Geometry check sheet. Reference: the model listing, model coordinates, mm. Face numbers are marked on the shaded views. A direction names the side the tool comes from. Give positions to 0.01 mm unless a question says otherwise; leave off trailing zeros. Order: outer loops, then holes, each group sorted by start corner. A loop starts at its lowest first (then second) coordinate and runs counter-clockwise, first axis right, second up. Notation, with made-up numbers: M -29.5,72 L -17.5,72 A20 cw -17.5,108 Z; hole C 26.25,-11.5 d3. An arc over 180 degrees is marked long. One line per question, with ' | ' between items. Start each with the question number.
from build123d import *

# Parameters (mm, degrees)
Y_KSEKLIK_EKSTR_ZYON4_DEPTH = 20
IZIM5_R                     = 67.8
IZIM5_R_2                   = 50
KES_EKSTR_ZYON1_DEPTH       = 10
IZIM7_R                     = 50
KES_EKSTR_ZYON2_DEPTH       = 20


with BuildPart() as part:
    # Çizim1 → Yükseklik-Ekstrüzyon4 (new body)
    with BuildSketch(Plane(origin=(0, 0, 0), x_dir=(1, 0, 0), z_dir=(0, 1, 0))):
        with BuildLine():
            ThreePointArc((-141.825379968, 39.155786128), (-171.116823462, 33.971749541), (-188.729833462, 10))
            Line((-188.729833462, 10), (-172.912878475, 10))
            ThreePointArc((-172.912878475, 10), (-125, 0), (-172.912878475, -10))
            Line((-172.912878475, -10), (-188.729833462, -10))
            ThreePointArc((-188.729833462, -10), (-171.116823462, -33.971749541), (-141.825379968, -39.155786128))
            ThreePointArc((-141.825379968, -39.155786128), (-90.896626459, -39.380855183), (-44.495770634, -60.374882159))
            ThreePointArc((-44.495770634, -60.374882159), (0, -75), (44.495770634, -60.374882159))
            ThreePointArc((44.495770634, -60.374882159), (90.896626459, -39.380855183), (141.825379968, -39.155786128))
            ThreePointArc((141.825379968, -39.155786128), (171.116823462, -33.971749541), (188.729833462, -10))
            Line((188.729833462, -10), (172.912878475, -10))
            ThreePointArc((172.912878475, -10), (125, 0), (172.912878475, 10))
            Line((172.912878475, 10), (188.729833462, 10))
            ThreePointArc((188.729833462, 10), (171.116823462, 33.971749541), (141.825379968, 39.155786128))
            ThreePointArc((141.825379968, 39.155786128), (90.896626459, 39.380855183), (44.495770634, 60.374882159))
            ThreePointArc((44.495770634, 60.374882159), (0, 75), (-44.495770634, 60.374882159))
            ThreePointArc((-44.495770634, 60.374882159), (-90.896626459, 39.380855183), (-141.825379968, 39.155786128))
        make_face()
    extrude(amount=Y_KSEKLIK_EKSTR_ZYON4_DEPTH)

    # Çizim5 → Kes-Ekstrüzyon1 (cut)
    with BuildSketch(Plane(origin=(0, 20, 0), x_dir=(1, 0, 0), z_dir=(0, 1, 0))):
        with Locations(Location((0, 0, 0), (0, 0, 270))):
            Circle(IZIM5_R)
        with Locations(Location((0, 0, 0), (0, 0, 270))):
            Circle(IZIM5_R_2, mode=Mode.SUBTRACT)
    extrude(amount=-KES_EKSTR_ZYON1_DEPTH, mode=Mode.SUBTRACT)

    # Çizim7 → Kes-Ekstrüzyon2 (cut)
    with BuildSketch(Plane(origin=(0, 20, 0), x_dir=(1, 0, 0), z_dir=(0, 1, 0))):
        with Locations(Location((0, 0, 0), (0, 0, 270))):
            Circle(IZIM7_R)
    extrude(amount=-KES_EKSTR_ZYON2_DEPTH, mode=Mode.SUBTRACT)


solid = part.part
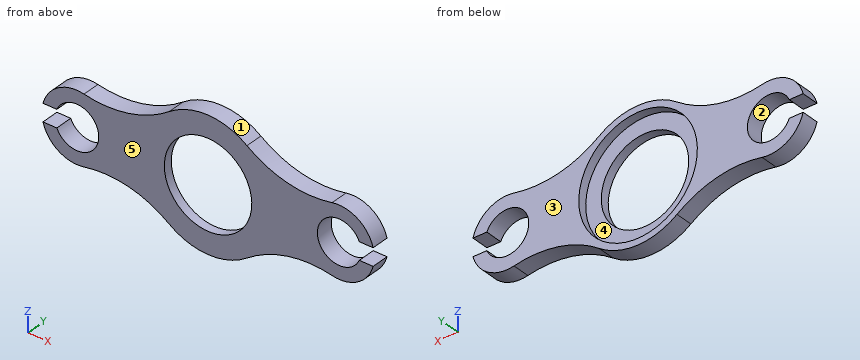
Item 1: Cross-section at A-A, the plane x = 0. Record the cut outline in (y, z), plus the area to 3 significant figures.
Item 2: Cross-section at D-D, the plane x = 150. Record the cut outline in (y, z).
Item 3: Material ranges on line 1 along X through (y, z) = (14, 0); line 2 along X through (y, z) = (9, 0); line 3 along X through (y, z) = (10.5, 16.5), recorded low to high.
Item 4: Mould release check, pull along X, two halves, no side actions. Record for the marked faces 1, 2 and 3: released by +X, released by -X, zero draft, split by the parting line, or undercut.
Item 5: Cross-section at B-B, the plane z = 0. Record the cut outline in (x, y).
Item 6: Cross-section at C-C, the plane z = 21. Record the cut outline in (x, y).
Item 7: Depth check by flat-ended pin: pin 1 (3 mm diameter, centred on x = 64, y = 12.5, fed in from -Z); pin 2 (1.5 mm diameter, centred on x = 122, y = 7, fed in from -Z); pin 3 (2 mm diameter, centred on y = 6, z = 37, fed in from -X). Enter the tip coordinate at first touch or a pass-through.
Item 8: Set-up check for the marked faces 4 and 5: record each of +Z, -Z, +X, -X, +Y, -Y from which the full face is reachable in a straight line by a thin tool's end or side.
Outcome:
1) outline: M 0,-75 L 20,-75 L 20,-67.8 L 10,-67.8 L 10,-50 L 0,-50 Z; M 0,50 L 10,50 L 10,67.8 L 20,67.8 L 20,75 L 0,75 Z | area: 644 mm²
2) outline: M 0,-40 L 20,-40 L 20,-25 L 0,-25 Z; M 0,25 L 20,25 L 20,40 L 0,40 Z
3) line 1: x = -125 to -67.8, 67.8 to 125 | line 2: x = -125 to -50, 50 to 125 | line 3: x = -186.44 to -168.78, -131.22 to -65.76, 65.76 to 131.22, 168.78 to 186.44
4) face 1: split by the parting line | face 2: undercut | face 3: zero draft
5) outline: M -125,0 L -50,0 L -50,10 L -67.8,10 L -67.8,20 L -125,20 Z; M 50,0 L 125,0 L 125,20 L 67.8,20 L 67.8,10 L 50,10 Z
6) outline: M -184.04,0 L -163.56,0 L -163.56,20 L -184.04,20 Z; M -136.44,0 L -45.38,0 L -45.38,10 L -64.47,10 L -64.47,20 L -136.44,20 Z; M 45.38,0 L 136.44,0 L 136.44,20 L 64.47,20 L 64.47,10 L 45.38,10 Z; M 163.56,0 L 184.04,0 L 184.04,20 L 163.56,20 Z
7) pin 1: stops at z = -49.37 | pin 2: stops at z = -36.72 | pin 3: stops at x = -167.44
8) face 4: +Y | face 5: +Z, -Z, +X, -X, -Y
